Here's the drawing with two shaded views (mm, measured from the low corner). I have some questions. A direction names the side the tool comes from. Give positions to 0.01 mm unless a question says otherwise; leave off trailing zeros. Loops run counter-clockwise (first coordinate to the right, second up) from the corner with the lowest first, then second, coordinate; pieces in that order, holes last. Notation, with made-up numbers: M 61,41 L 65,41 A21 cw 65,52 Z; hole C 19,-36.5 d7. An arc over 180 degrees is marked long. Put each result on its own line as item: value. Start each with the question number.
1) Please list where these lines run through material, in increasing order: line 1 along X through (y, z) = (20.5, 34.5); line 2 along Y through (x, z) = (49, 11). Write a range as from..to.
2) For P1, Ø10, axis at y = 39.5, z = 13.5, coming from the +X side (3 decimals); P2, Ø4, axis at x = 82, y = 18.5, coming from the +Z side; P3, Ø8, axis at x = 92, z = 6, coming from the +Y side, each with a flat end and sliding along its axis, tell me the tip position at first contact or that it passes through.
3) Imagine slicing it at B-B (y = 34). Write out the boundary of the cut face in (x, z) (3 decimals).
4) If we mould it in two halves opening along X, with no side actions, what happens to the marked faces 6, 7, 8 and 9? For each: +X half, -X half, draft (parallel to the pull), parting line (faces both ways), or undercut.
5) For the marked faces 1, 2, 3, 4 and 5, which set-ups out of +Z, -Z, +X, -X, +Y, -Y let a thin tool reach every point of the face, with its end or its side?
6) Imagine slicing it at A-A (z = 16). Write out the boundary of the cut face in (x, y) (3 decimals), then the cut area to 3 significant figures.
7) Imagine slicing it at D-D (x = 15). Write out the boundary of the cut face in (y, z), then the cut area to 3 significant figures.
8) Imagine slicing it at C-C (x = 33). Write out the boundary of the cut face in (y, z), then the cut area to 3 significant figures.
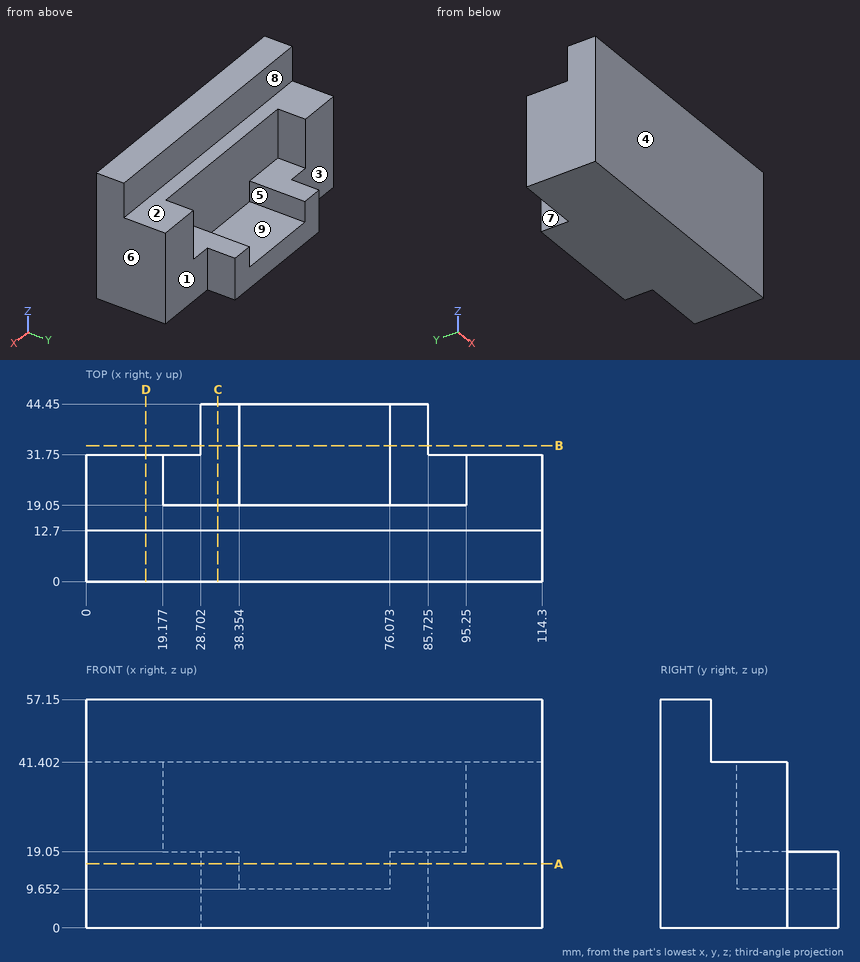
Recorded:
1. line 1: 0..19.18, 95.25..114.3
1. line 2: 0..19.05
2. P1: x = 85.725
2. P2: z = 41.4
2. P3: y = 31.75
3. outline: M 28.702,0 L 85.725,0 L 85.725,19.05 L 76.073,19.05 L 76.073,9.652 L 38.354,9.652 L 38.354,19.05 L 28.702,19.05 Z
4. face 6: +X half
4. face 7: -X half
4. face 8: draft
4. face 9: undercut
5. face 1: +Z, -Z, +X, +Y
5. face 2: +Z, +X, -X, +Y
5. face 3: +Z, -Z, -X, +Y
5. face 4: +Z, -Z, +X, -X, -Y
5. face 5: +Z, +Y
6. outline: M 0,0 L 114.3,0 L 114.3,31.75 L 85.725,31.75 L 85.725,44.45 L 76.073,44.45 L 76.073,19.05 L 38.354,19.05 L 38.354,44.45 L 28.702,44.45 L 28.702,31.75 L 0,31.75 Z
6. area: 3,400 mm²
7. outline: M 0,0 L 31.75,0 L 31.75,41.4 L 12.7,41.4 L 12.7,57.15 L 0,57.15 Z
7. area: 1,510 mm²
8. outline: M 0,0 L 44.45,0 L 44.45,19.05 L 19.05,19.05 L 19.05,41.4 L 12.7,41.4 L 12.7,57.15 L 0,57.15 Z
8. area: 1,470 mm²
